from build123d import *

# Parameters (mm, degrees)
SKETCH1_W                = 20
SKETCH1_H                = 80
BOSS_EXTRUDE1_DEPTH      = 40
BOSS_EXTRUDE1_2_DEPTH    = 40
BOSS_EXTRUDE2_START      = -20
BOSS_EXTRUDE2_DEPTH      = 20
BOSS_EXTRUDE3_START      = -20
BOSS_EXTRUDE3_DEPTH      = 20
SKETCH5_R                = 10
CUT_EXTRUDE2_DEPTH       = 170
FILLET2_R                = 5
FILLET3_R                = 5
BOSS_EXTRUDE4_DEPTH      = 50
BOSS_EXTRUDE4_DEPTH_BACK = 190
SKETCH6_R                = 10
SKETCH10_R               = 19
BOSS_EXTRUDE6_DEPTH      = 5
SKETCH11_R               = 15
BOSS_EXTRUDE7_DEPTH      = 100


with BuildPart() as part:
    # Sketch1 → Boss-Extrude1 (new body)
    with BuildSketch(Plane(origin=(0, 0, 0), x_dir=(1, 0, 0), z_dir=(0, 1, 0))):
        with Locations((70, 0)):
            Rectangle(SKETCH1_W, SKETCH1_H)
    extrude(amount=BOSS_EXTRUDE1_DEPTH)

    # Sketch4 → Boss-Extrude3 (add)
    with BuildSketch(Plane(origin=(80, 0, 0), x_dir=(0, 0, -1), z_dir=(1, 0, 0)).offset(BOSS_EXTRUDE3_START)):
        with BuildLine():
            Line((-25, 50), (-25, 40))
            Line((-25, 40), (25, 40))
            Line((25, 40), (25, 50))
            ThreePointArc((25, 50), (0, 75), (-25, 50))
        make_face()
    extrude(amount=BOSS_EXTRUDE3_DEPTH)


with BuildPart() as body_2:
    # Sketch1 → Boss-Extrude1 2 (new body)
    with BuildSketch(Plane(origin=(0, 0, 0), x_dir=(1, 0, 0), z_dir=(0, 1, 0))):
        with Locations((-70, 0)):
            Rectangle(SKETCH1_W, SKETCH1_H)
    extrude(amount=BOSS_EXTRUDE1_2_DEPTH)

    # Sketch2 → Boss-Extrude2 (add)
    with BuildSketch(Plane.ZY.offset(80).offset(BOSS_EXTRUDE2_START)):
        with BuildLine():
            Line((-25, 50), (-25, 40))
            Line((-25, 40), (25, 40))
            Line((25, 40), (25, 50))
            ThreePointArc((25, 50), (0, 75), (-25, 50))
        make_face()
    extrude(amount=BOSS_EXTRUDE2_DEPTH)


with BuildPart() as cut_extrude2_tool:
    # Sketch5 → Cut-Extrude2 (new body)
    with BuildSketch(Plane.ZY.offset(80)):
        with Locations((0, 50)):
            Circle(SKETCH5_R)
    extrude(amount=-CUT_EXTRUDE2_DEPTH)


with BuildPart() as part_1:
    add(part.part)

    # Cut-Extrude2: cut by cut_extrude2_tool
    add(cut_extrude2_tool.part, mode=Mode.SUBTRACT)

    # Fillet3
    fillet3_edges = [part_1.edges().sort_by_distance(p)[0] for p in [
        (70, 40, -25),
        (70, 40, 25),
    ]]
    fillet(fillet3_edges, radius=FILLET3_R)



with BuildPart() as body_2_1:
    add(body_2.part)

    # Cut-Extrude2: cut by cut_extrude2_tool
    add(cut_extrude2_tool.part, mode=Mode.SUBTRACT)

    # Fillet2
    fillet2_edges = [body_2_1.edges().sort_by_distance(p)[0] for p in [
        (-70, 40, 25),
        (-70, 40, -25),
    ]]
    fillet(fillet2_edges, radius=FILLET2_R)


with BuildPart() as part_2:
    add(part_1.part)

    add(body_2_1.part)  # Boss-Extrude4 merges body 2
    # Sketch6 → Boss-Extrude4 (add, two sides: drawn at the far end of the back side and taken through both)
    with BuildSketch(Plane.ZY.offset(80).offset(-BOSS_EXTRUDE4_DEPTH_BACK)):
        with Locations((0, 50)):
            Circle(SKETCH6_R)
    extrude(amount=BOSS_EXTRUDE4_DEPTH + BOSS_EXTRUDE4_DEPTH_BACK)

    # Sketch10 → Boss-Extrude6 (add)
    with BuildSketch(Plane(origin=(-50, 0, 0), x_dir=(0, 0, -1), z_dir=(1, 0, 0))):
        with Locations((0, 50)):
            Circle(SKETCH10_R)
    boss_extrude6 = extrude(amount=BOSS_EXTRUDE6_DEPTH)

    # Mirror9: Boss-Extrude6 across plane
    add(boss_extrude6.mirror(Plane(origin=(0, 0, 0), x_dir=(0, 0, 1), z_dir=(1, 0, 0))))

    # Sketch11 → Boss-Extrude7 (add)
    with BuildSketch(Plane(origin=(-50, 0, 0), x_dir=(0, 0, -1), z_dir=(1, 0, 0))):
        with Locations(Location((0, 50, 0), (0, 0, 180))):
            Circle(SKETCH11_R)
    extrude(amount=BOSS_EXTRUDE7_DEPTH)


solid = part_2.part
Source: CAD feature listing. Evaluate the final solid. Frame: model axes, mm. A direction names the side the tool comes from. Round coordinates to 2 decimals unless told otherwise and drop trailing zeros. Loops run counter-clockwise (first coordinate to the right, second up) from the corner with the lowest first, then second, coordinate; pieces in that order, holes last. Notation, with made-up numbers: M -13,-35.75 L -5,-35.75 A27 cw -5,-1.75 Z; hole C 21.5,38.5 d5. An arc over 180 degrees is marked long. Return JSON: item names as keys, results as strings. Group by question number.
1. Material intervals for line 1 along X through (y, z) = (31.5, -2); line 2 along X through (y, z) = (62, 8.5); line 3 along X through (y, z) = (6, -23.5), sorted ascending. Write a range as from..to.
2. Pin query (flat end, axial travel): pin 1 (5.5 mm diameter, centred on x = -75, y = 46.5, fed in from -Z); pin 2 (11 mm diameter, centred on x = -70, z = 34, fed in from +Y); pin 3 (1 mm diameter, centred on x = -58.5, z = 5, fed in from -Y). Return the tip coordinate at first contact, or that it passes through.
3. Section query A-A on y = 62.5. Output: boundary loops of the cut face in (x, z).
4. Section query C-C on x = -23.5. Output: boundary loops of the cut face in (y, z).
5. Section query B-B on x = 54.5. Output: boundary loops of the cut face in (y, z).
6. Reachability of faces 1 (the face through (70, 47, -25)), 2 (the face through (-104.65, 40.24, -2.17)), 3 (the face through (-50, 42, -8)), 4 (the face through (70, 48, 25)) from +Z, -Z, +X, -X, +Y, -Y: full face, straight path, thin tool, end or side. Return the list, or none.
7. Mould query, pull axis X, two halves, no side actions, for faces 5 (the face through (-80, 29, 1)), 6 (the face through (70, 41, 27)), 7 (the face through (45, 56, -14)). Classes: released by +X, released by -X, zero draft, split by the parting line, or undercut.
Checks:
{
 "1": {"line 1": "x = -80..-60, -50..-45, 45..50, 60..80", "line 2": "x = -80..-60, -50..50, 60..80", "line 3": "x = -80..-60, 60..80"},
 "2": {"pin 1": "stops at z = -25.16", "pin 2": "stops at y = 40.23", "pin 3": "stops at y = 41.07"},
 "3": {"outline": "M -80,-21.65 L -60,-21.65 L -60,21.65 L -80,21.65 Z; M -50,-14.31 L -45,-14.31 L -45,-8.29 L 45,-8.29 L 45,-14.31 L 50,-14.31 L 50,14.31 L 45,14.31 L 45,8.29 L -45,8.29 L -45,14.31 L -50,14.31 Z; M 60,-21.65 L 80,-21.65 L 80,21.65 L 60,21.65 Z"},
 "4": {"outline": "C 50,0 d30"},
 "5": {"outline": "C 50,0 d20"},
 "6": {"face 1": "-Z, +X, -X, +Y", "face 2": "-X", "face 3": "none", "face 4": "+Z, +X, -X, +Y"},
 "7": {"face 5": "released by -X", "face 6": "zero draft", "face 7": "undercut"}
}
